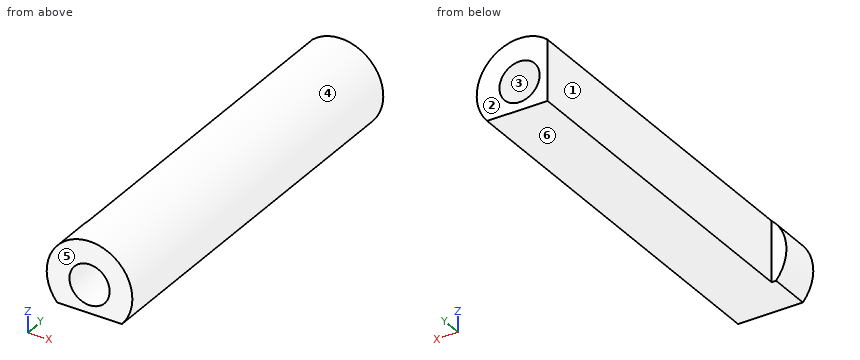
from build123d import *

# Parameters (mm, degrees)
SKETCH1_R           = 4.9
SKETCH1_R_2         = 2.3
BOSS_EXTRUDE1_DEPTH = 44.8
SKETCH2_W           = 12.911728521
SKETCH2_H           = 2.871421643
CUT_EXTRUDE1_DEPTH  = 45
SKETCH3_W           = 17.671201811
SKETCH3_H           = 20
CUT_EXTRUDE2_DEPTH  = 40


with BuildPart() as part:
    # Sketch1 → Boss-Extrude1 (new body)
    with BuildSketch(Plane(origin=(0, 0, 0), x_dir=(1, 0, 0), z_dir=(0, 1, 0))):
        with Locations(Location((0, 0, 0), (0, 0, 270))):
            Circle(SKETCH1_R)
        with Locations(Location((0, 0, 0), (0, 0, 270))):
            Circle(SKETCH1_R_2, mode=Mode.SUBTRACT)
    extrude(amount=BOSS_EXTRUDE1_DEPTH)

    # Sketch2 → Cut-Extrude1 (cut)
    with BuildSketch(Plane(origin=(0, 44.8, 0), x_dir=(1, 0, 0), z_dir=(0, 1, 0))):
        with Locations((0.901888867, 4.635710822)):
            Rectangle(SKETCH2_W, SKETCH2_H)
    extrude(amount=-CUT_EXTRUDE1_DEPTH, mode=Mode.SUBTRACT)

    # Sketch3 → Cut-Extrude2 (cut)
    with BuildSketch(Plane(origin=(0, 44.8, 0), x_dir=(1, 0, 0), z_dir=(0, 1, 0))):
        with Locations((-12.035600906, 4.200665125)):
            Rectangle(SKETCH3_W, SKETCH3_H)
    extrude(amount=-CUT_EXTRUDE2_DEPTH, mode=Mode.SUBTRACT)


solid = part.part
Design review of the part built by this model. Coordinates are the model's own, in mm. Face numbers are marked on the shaded views. A direction names the side the tool comes from. Round coordinates to 2 decimals unless told otherwise and drop trailing zeros. Write each loop counter-clockwise with the first axis right and the second up, starting at its lowest first coordinate (ties: lowest second). Pieces come first, ordered by that corner, then holes. Notation, with made-up numbers: M -12.5,35.5 L 46.5,35.5 A21 cw 46.5,67.5 Z; hole C -5,-33.75 d8. An arc over 180 degrees is marked long. One line per item, written item: value. Start each with the question number.
1. To check wall thickness, follow probe 1 along X at (y, z) = (21, 0); probe 2 along X at (y, z) = (27, 0.5) (3 decimals); probe 3 along Z at (x, y) = (-1.25, 38.5). State the ranges of each line that lie inside material, in increasing order. Write a range as from..to.
2. Clearance check with flat-ended pins moving along their axes: P1, Ø2, axis at x = -2.5, y = 13.5, coming from the +Z side; P2, Ø0.8, axis at x = -4, z = 0.5, coming from the +Y side. State where each tip first meets the part, or that it passes through.
3. Take a section at A-A on x = 0. State the section outline as (y, z) points, then the cut area to 3 significant figures.
4. Take a section at C-C on y = 9. State the section outline as (x, z) points.
5. Take a section at B-B on z = 0. State the section outline as (x, y) points.
6. Take a section at D-D on z = 1.75. State the section outline as (x, y) points, then the cut area to 3 significant figures.
7. For the marked faces 1 and 2, list the 3-axis set-ups (+Z, -Z, +X, -X, +Y, -Y) from which the entire face can be reached by the end or side of a thin tool; tool diameter is ignored.
8. Draft analysis for pull direction Z (two halves, no side actions). For the marked faces 3, 4, 5 and 6, state which applies: pulls with the +Z half, pulls with the -Z half, needs draft (parallel to the pull), parting line crosses it, or undercut.
Computed:
1. probe 1: x = -3.2..-2.3, 2.3..4.9
1. probe 2: x = -3.2..-2.245, 2.245..4.874
1. probe 3: z = -3.2..-1.93, 1.93..4.74
2. P1: stops at z = 4.66
2. P2: stops at y = 4.8
3. outline: M 0,-3.2 L 44.8,-3.2 L 44.8,-2.3 L 0,-2.3 Z; M 0,2.3 L 44.8,2.3 L 44.8,4.9 L 0,4.9 Z
3. area: 157 mm²
4. outline: M -3.2,-3.2 L 3.71,-3.2 A4.9 ccw -3.2,3.71 Z; hole C 0,0 d4.6
5. outline: M -4.9,0 L -2.3,0 L -2.3,44.8 L -3.2,44.8 L -3.2,4.8 L -4.9,4.8 Z; M 2.3,0 L 4.9,0 L 4.9,44.8 L 2.3,44.8 Z
6. outline: M -4.58,0 L -1.49,0 L -1.49,44.8 L -3.2,44.8 L -3.2,4.8 L -4.58,4.8 Z; M 1.49,0 L 4.58,0 L 4.58,44.8 L 1.49,44.8 Z
6. area: 221 mm²
7. face 1: +Z, -Z, -X, +Y
7. face 2: +Z, -Z, +X, -X, +Y
8. face 3: undercut
8. face 4: parting line crosses it
8. face 5: needs draft
8. face 6: pulls with the -Z half
